Check sheet for the modelled part. Datum: model origin and axes. Units: mm. Face numbers are marked on the shaded views. A direction names the side the tool comes from. Coordinates: 2 decimals unless noted, no trailing zeros. Loops run counter-clockwise (first coordinate to the right, second up) from the corner with the lowest first, then second, coordinate; pieces in that order, holes last.
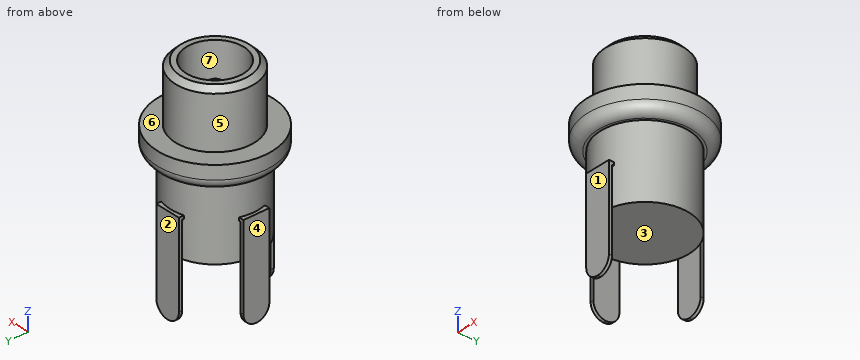
Autodesk Inventor part; units mm, degrees
ref_plane "YZ Plane" through (0, 0, 0) normal (1, 0, 0) x (0, 1, 0)
ref_plane "XZ Plane" through (0, 0, 0) normal (0, 1, 0) x (-1, 0, 0)
ref_plane "XY Plane" through (0, 0, 0) normal (0, 0, 1) x (1, 0, 0)
sketch "Esquisse1" plane through (0, 0, 0) normal (0, 0, 1) x (1, 0, 0)
  circle A0 centre (0, 0) radius 3.775
  dimension "d0" = 7.55
extrude "Extrusion1" add sketch "Esquisse1" along normal blind 5.5
sketch "Esquisse2" plane through (0, 0, 0) normal (0, 0, -1) x (-1, 0, 0)
  circle A0 centre (0, 0) radius 5.5
  dimension "d3" = 11
extrude "Extrusion2" add sketch "Esquisse2" along normal blind 2.3
sketch "Esquisse3" plane through (0, 0, -2.3) normal (0, 0, -1) x (-1, 0, 0)
  circle A0 centre (0, 0) radius 4.25
  dimension "d6" = 8.5
extrude "Extrusion3" add sketch "Esquisse3" along normal blind 7
fillet "Congé1" radius 1 1 edges at (5.5, 0, -2.3)
sketch "Esquisse4" plane through (0, 0, 5.5) normal (0, 0, 1) x (1, 0, 0)
  circle A0 centre (0, 0) radius 2.75
  dimension "d10" = 5.5
extrude "Extrusion4" cut sketch "Esquisse4" against normal blind 9
sketch "Esquisse5" plane through (0, 0, -3.5) normal (0, 0, 1) x (1, 0, 0)
  circle A0 centre (0, 0) radius 1.2
  dimension "d13" = 2.4
extrude "Extrusion5" add sketch "Esquisse5" along normal blind 7.2
fillet "Congé2" radius 1.2 1 edges at (-1.2, 0, 3.7)
thread "Filetage1"
sketch "Esquisse6" plane through (0, 0, 0) normal (1, 0, 0) x (0, 1, 0)
  line L0 (4.25, -14.8) -> (4.25, -5.8)
  line L1 (4.25, -5.8) -> (4.05, -5.8)
  line L2 (4.05, -5.8) -> (4.05, -5.5)
  line L3 (4.05, -5.5) -> (4.55, -5.5)
  line L4 (4.55, -5.5) -> (4.55, -14.8)
  line L5 (4.55, -14.8) -> (4.25, -14.8)
  line L6 (4.25, -2.3) -> (4.25, -9.3)
  line L7 (4.25, -2.3) -> (-4.25, -2.3)
  point P0 (0, 0)
  dimension "d19" = 0.3
  dimension "d20" = 0.3
  dimension "d21" = 9.3
  dimension "d22" = 3.2
  dimension "d24" = 0.2
extrude "Extrusion6" add sketch "Esquisse6" along normal mid plane 2.5
fillet "Congé3" radius 1.25 2 edges at (1.25, 4.4, -14.8) (-1.25, 4.4, -14.8)
pattern_circular "Réseau circulaire1" count 3 over 180 about axis through (0, 0, -10) along (0, 0, 1) of "Extrusion6", "Congé3"
chamfer "Chanfrein1" distance 0.5 angle 45 1 edges at (-3.775, 0, 5.5)
properties part number "Plug alimentation" material "----------"
1) Scan lines: line 1 (Y direction, x = 0, z = -0.75); line 2 (X direction, y = -0.5, z = -12); line 3 (Z direction, x = -0.5, y = -4). Record each from-to range of solid material in increasing order.
Answer sheet:
line 1: y = -5.5 to -2.75, -1.2 to 1.2, 2.75 to 5.5
line 2: x = -4.55 to -4.25
line 3: z = -9.3 to 0
2) Depth check by flat-ended pin: pin 1 (0.8 mm diameter, centred on y = -0.5, z = -11.5, fed in from +X); pin 2 (3 mm diameter, centred on y = 1, z = -3, fed in from +X); pin 3 (1 mm diameter, centred on x = -1.5, z = 1.5, fed in from +Y). Enter the tip coordinate at first touch or a pass-through.
Answer sheet:
pin 1: stops at x = -4.25
pin 2: stops at x = 5.44
pin 3: stops at y = 3.64
3) Mould release check, pull along X, two halves, no side actions. Record for the marked faces 4, 5, 6 and 7: +X half, -X half, draft (parallel to the pull), parting line (faces both ways), or undercut.
Answer sheet:
face 4: -X half
face 5: parting line
face 6: draft
face 7: undercut
4) Set-up check for the marked faces 1, 2 and 3: record each of +Z, -Z, +X, -X, +Y, -Y from which the full face is reachable in a straight line by a thin tool's end or side.
Answer sheet:
face 1: -Z, +X, -X, -Y
face 2: -Z, +X, -X, +Y
face 3: -Z, +X
5) Section check A-A on z = 2. Enter the section's corners in (x, y) (3 decimals), plus the area to 3 significant figures.
Answer sheet:
outline: circle Ø7.55 at (0, 0); circle Ø2.4 at (0, 0); hole circle Ø5.5 at (0, 0)
area: 25.5 mm2
